```python
from build123d import *

# Parameters (mm, degrees)
BOSS_EXTRUDE1_DEPTH = 2
SKETCH2_R           = 1.5
CUT_EXTRUDE1_DEPTH  = 83.048765987
SKETCH3_R           = 1
CUT_EXTRUDE2_DEPTH  = 83.048765987


with BuildPart() as part:
    # Sketch1 → Boss-Extrude1 (new body)
    with BuildSketch(Plane(origin=(0, 0, 0), x_dir=(1, 0, 0), z_dir=(0, 1, 0))):
        with BuildLine():
            Line((53, 58), (-53, 58))
            ThreePointArc((-53, 58), (-56.535533906, 56.535533906), (-58, 53))
            Line((-58, 53), (-58, -53))
            ThreePointArc((-58, -53), (-56.535533906, -56.535533906), (-53, -58))
            Line((-53, -58), (53, -58))
            ThreePointArc((53, -58), (56.535533906, -56.535533906), (58, -53))
            Line((58, -53), (58, 53))
            ThreePointArc((58, 53), (56.535533906, 56.535533906), (53, 58))
        make_face()
    extrude(amount=BOSS_EXTRUDE1_DEPTH)

    # Sketch2 → Cut-Extrude1 (cut, through all)
    with BuildSketch(Plane(origin=(0, 2, 0), x_dir=(1, 0, 0), z_dir=(0, 1, 0))):
        with Locations(Location((-45.60494968, 43.386330507, 0), (0, 0, 270))):
            Circle(SKETCH2_R)
        with Locations(Location((-35.60494968, 43.386330507, 0), (0, 0, 270))):
            Circle(SKETCH2_R)
        with Locations(Location((-25.60494968, 43.386330507, 0), (0, 0, 270))):
            Circle(SKETCH2_R)
        with Locations(Location((-15.60494968, 43.386330507, 0), (0, 0, 270))):
            Circle(SKETCH2_R)
        with Locations(Location((-5.60494968, 43.386330507, 0), (0, 0, 270))):
            Circle(SKETCH2_R)
        with Locations(Location((4.39505032, 43.386330507, 0), (0, 0, 270))):
            Circle(SKETCH2_R)
        with Locations(Location((14.39505032, 43.386330507, 0), (0, 0, 270))):
            Circle(SKETCH2_R)
        with Locations(Location((24.39505032, 43.386330507, 0), (0, 0, 270))):
            Circle(SKETCH2_R)
        with Locations(Location((34.39505032, 43.386330507, 0), (0, 0, 270))):
            Circle(SKETCH2_R)
        with Locations(Location((44.39505032, 43.386330507, 0), (0, 0, 270))):
            Circle(SKETCH2_R)
        with Locations(Location((-35.60494968, 33.386330507, 0), (0, 0, 270))):
            Circle(SKETCH2_R)
        with Locations(Location((-25.60494968, 33.386330507, 0), (0, 0, 270))):
            Circle(SKETCH2_R)
        with Locations(Location((-15.60494968, 33.386330507, 0), (0, 0, 270))):
            Circle(SKETCH2_R)
        with Locations(Location((-5.60494968, 33.386330507, 0), (0, 0, 270))):
            Circle(SKETCH2_R)
        with Locations(Location((4.39505032, 33.386330507, 0), (0, 0, 270))):
            Circle(SKETCH2_R)
        with Locations(Location((14.39505032, 33.386330507, 0), (0, 0, 270))):
            Circle(SKETCH2_R)
        with Locations(Location((24.39505032, 33.386330507, 0), (0, 0, 270))):
            Circle(SKETCH2_R)
        with Locations(Location((34.39505032, 33.386330507, 0), (0, 0, 270))):
            Circle(SKETCH2_R)
        with Locations(Location((44.39505032, 33.386330507, 0), (0, 0, 270))):
            Circle(SKETCH2_R)
        with Locations(Location((-35.60494968, 23.386330507, 0), (0, 0, 270))):
            Circle(SKETCH2_R)
        with Locations(Location((-25.60494968, 23.386330507, 0), (0, 0, 270))):
            Circle(SKETCH2_R)
        with Locations(Location((-15.60494968, 23.386330507, 0), (0, 0, 270))):
            Circle(SKETCH2_R)
        with Locations(Location((-5.60494968, 23.386330507, 0), (0, 0, 270))):
            Circle(SKETCH2_R)
        with Locations(Location((4.39505032, 23.386330507, 0), (0, 0, 270))):
            Circle(SKETCH2_R)
        with Locations(Location((14.39505032, 23.386330507, 0), (0, 0, 270))):
            Circle(SKETCH2_R)
        with Locations(Location((24.39505032, 23.386330507, 0), (0, 0, 270))):
            Circle(SKETCH2_R)
        with Locations(Location((34.39505032, 23.386330507, 0), (0, 0, 270))):
            Circle(SKETCH2_R)
        with Locations(Location((44.39505032, 23.386330507, 0), (0, 0, 270))):
            Circle(SKETCH2_R)
        with Locations(Location((-35.60494968, 13.386330507, 0), (0, 0, 270))):
            Circle(SKETCH2_R)
        with Locations(Location((-25.60494968, 13.386330507, 0), (0, 0, 270))):
            Circle(SKETCH2_R)
        with Locations(Location((-15.60494968, 13.386330507, 0), (0, 0, 270))):
            Circle(SKETCH2_R)
        with Locations(Location((-5.60494968, 13.386330507, 0), (0, 0, 270))):
            Circle(SKETCH2_R)
        with Locations(Location((4.39505032, 13.386330507, 0), (0, 0, 270))):
            Circle(SKETCH2_R)
        with Locations(Location((14.39505032, 13.386330507, 0), (0, 0, 270))):
            Circle(SKETCH2_R)
        with Locations(Location((24.39505032, 13.386330507, 0), (0, 0, 270))):
            Circle(SKETCH2_R)
        with Locations(Location((34.39505032, 13.386330507, 0), (0, 0, 270))):
            Circle(SKETCH2_R)
        with Locations(Location((44.39505032, 13.386330507, 0), (0, 0, 270))):
            Circle(SKETCH2_R)
        with Locations(Location((-35.60494968, 3.386330507, 0), (0, 0, 270))):
            Circle(SKETCH2_R)
        with Locations(Location((-25.60494968, 3.386330507, 0), (0, 0, 270))):
            Circle(SKETCH2_R)
        with Locations(Location((-15.60494968, 3.386330507, 0), (0, 0, 270))):
            Circle(SKETCH2_R)
        with Locations(Location((-5.60494968, 3.386330507, 0), (0, 0, 270))):
            Circle(SKETCH2_R)
        with Locations(Location((4.39505032, 3.386330507, 0), (0, 0, 270))):
            Circle(SKETCH2_R)
        with Locations(Location((14.39505032, 3.386330507, 0), (0, 0, 270))):
            Circle(SKETCH2_R)
        with Locations(Location((24.39505032, 3.386330507, 0), (0, 0, 270))):
            Circle(SKETCH2_R)
        with Locations(Location((34.39505032, 3.386330507, 0), (0, 0, 270))):
            Circle(SKETCH2_R)
        with Locations(Location((44.39505032, 3.386330507, 0), (0, 0, 270))):
            Circle(SKETCH2_R)
        with Locations(Location((-35.60494968, -6.613669493, 0), (0, 0, 270))):
            Circle(SKETCH2_R)
        with Locations(Location((-25.60494968, -6.613669493, 0), (0, 0, 270))):
            Circle(SKETCH2_R)
        with Locations(Location((-15.60494968, -6.613669493, 0), (0, 0, 270))):
            Circle(SKETCH2_R)
        with Locations(Location((-5.60494968, -6.613669493, 0), (0, 0, 270))):
            Circle(SKETCH2_R)
        with Locations(Location((4.39505032, -6.613669493, 0), (0, 0, 270))):
            Circle(SKETCH2_R)
        with Locations(Location((14.39505032, -6.613669493, 0), (0, 0, 270))):
            Circle(SKETCH2_R)
        with Locations(Location((24.39505032, -6.613669493, 0), (0, 0, 270))):
            Circle(SKETCH2_R)
        with Locations(Location((34.39505032, -6.613669493, 0), (0, 0, 270))):
            Circle(SKETCH2_R)
        with Locations(Location((44.39505032, -6.613669493, 0), (0, 0, 270))):
            Circle(SKETCH2_R)
        with Locations(Location((-35.60494968, -16.613669493, 0), (0, 0, 270))):
            Circle(SKETCH2_R)
        with Locations(Location((-25.60494968, -16.613669493, 0), (0, 0, 270))):
            Circle(SKETCH2_R)
        with Locations(Location((-15.60494968, -16.613669493, 0), (0, 0, 270))):
            Circle(SKETCH2_R)
        with Locations(Location((-5.60494968, -16.613669493, 0), (0, 0, 270))):
            Circle(SKETCH2_R)
        with Locations(Location((4.39505032, -16.613669493, 0), (0, 0, 270))):
            Circle(SKETCH2_R)
        with Locations(Location((14.39505032, -16.613669493, 0), (0, 0, 270))):
            Circle(SKETCH2_R)
        with Locations(Location((24.39505032, -16.613669493, 0), (0, 0, 270))):
            Circle(SKETCH2_R)
        with Locations(Location((34.39505032, -16.613669493, 0), (0, 0, 270))):
            Circle(SKETCH2_R)
        with Locations(Location((44.39505032, -16.613669493, 0), (0, 0, 270))):
            Circle(SKETCH2_R)
        with Locations(Location((-35.60494968, -26.613669493, 0), (0, 0, 270))):
            Circle(SKETCH2_R)
        with Locations(Location((-25.60494968, -26.613669493, 0), (0, 0, 270))):
            Circle(SKETCH2_R)
        with Locations(Location((-15.60494968, -26.613669493, 0), (0, 0, 270))):
            Circle(SKETCH2_R)
        with Locations(Location((-5.60494968, -26.613669493, 0), (0, 0, 270))):
            Circle(SKETCH2_R)
        with Locations(Location((4.39505032, -26.613669493, 0), (0, 0, 270))):
            Circle(SKETCH2_R)
        with Locations(Location((14.39505032, -26.613669493, 0), (0, 0, 270))):
            Circle(SKETCH2_R)
        with Locations(Location((24.39505032, -26.613669493, 0), (0, 0, 270))):
            Circle(SKETCH2_R)
        with Locations(Location((34.39505032, -26.613669493, 0), (0, 0, 270))):
            Circle(SKETCH2_R)
        with Locations(Location((44.39505032, -26.613669493, 0), (0, 0, 270))):
            Circle(SKETCH2_R)
        with Locations(Location((-35.60494968, -36.613669493, 0), (0, 0, 270))):
            Circle(SKETCH2_R)
        with Locations(Location((-25.60494968, -36.613669493, 0), (0, 0, 270))):
            Circle(SKETCH2_R)
        with Locations(Location((-15.60494968, -36.613669493, 0), (0, 0, 270))):
            Circle(SKETCH2_R)
        with Locations(Location((-5.60494968, -36.613669493, 0), (0, 0, 270))):
            Circle(SKETCH2_R)
        with Locations(Location((4.39505032, -36.613669493, 0), (0, 0, 270))):
            Circle(SKETCH2_R)
        with Locations(Location((14.39505032, -36.613669493, 0), (0, 0, 270))):
            Circle(SKETCH2_R)
        with Locations(Location((24.39505032, -36.613669493, 0), (0, 0, 270))):
            Circle(SKETCH2_R)
        with Locations(Location((34.39505032, -36.613669493, 0), (0, 0, 270))):
            Circle(SKETCH2_R)
        with Locations(Location((44.39505032, -36.613669493, 0), (0, 0, 270))):
            Circle(SKETCH2_R)
        with Locations(Location((-35.60494968, -46.613669493, 0), (0, 0, 270))):
            Circle(SKETCH2_R)
        with Locations(Location((-25.60494968, -46.613669493, 0), (0, 0, 270))):
            Circle(SKETCH2_R)
        with Locations(Location((-15.60494968, -46.613669493, 0), (0, 0, 270))):
            Circle(SKETCH2_R)
        with Locations(Location((-5.60494968, -46.613669493, 0), (0, 0, 270))):
            Circle(SKETCH2_R)
        with Locations(Location((4.39505032, -46.613669493, 0), (0, 0, 270))):
            Circle(SKETCH2_R)
        with Locations(Location((14.39505032, -46.613669493, 0), (0, 0, 270))):
            Circle(SKETCH2_R)
        with Locations(Location((24.39505032, -46.613669493, 0), (0, 0, 270))):
            Circle(SKETCH2_R)
        with Locations(Location((34.39505032, -46.613669493, 0), (0, 0, 270))):
            Circle(SKETCH2_R)
        with Locations(Location((44.39505032, -46.613669493, 0), (0, 0, 270))):
            Circle(SKETCH2_R)
        with Locations(Location((-45.60494968, 33.386330507, 0), (0, 0, 270))):
            Circle(SKETCH2_R)
        with Locations(Location((-45.60494968, 23.386330507, 0), (0, 0, 270))):
            Circle(SKETCH2_R)
        with Locations(Location((-45.60494968, 13.386330507, 0), (0, 0, 270))):
            Circle(SKETCH2_R)
        with Locations(Location((-45.60494968, 3.386330507, 0), (0, 0, 270))):
            Circle(SKETCH2_R)
        with Locations(Location((-45.60494968, -6.613669493, 0), (0, 0, 270))):
            Circle(SKETCH2_R)
        with Locations(Location((-45.60494968, -16.613669493, 0), (0, 0, 270))):
            Circle(SKETCH2_R)
        with Locations(Location((-45.60494968, -26.613669493, 0), (0, 0, 270))):
            Circle(SKETCH2_R)
        with Locations(Location((-45.60494968, -36.613669493, 0), (0, 0, 270))):
            Circle(SKETCH2_R)
        with Locations(Location((-45.60494968, -46.613669493, 0), (0, 0, 270))):
            Circle(SKETCH2_R)
    extrude(amount=-CUT_EXTRUDE1_DEPTH, mode=Mode.SUBTRACT)

    # Sketch3 → Cut-Extrude2 (cut, through all)
    with BuildSketch(Plane.XZ):
        with Locations(Location((-53, 53, 0), (0, 0, 270))):
            Circle(SKETCH3_R)
        with Locations(Location((53, -53, 0), (0, 0, 270))):
            Circle(SKETCH3_R)
    extrude(amount=-CUT_EXTRUDE2_DEPTH, mode=Mode.SUBTRACT)


solid = part.part
```
The listing builds one solid part. Answer for the finished solid, in the listing's coordinates (mm). Give positions to 0.01 mm unless a question says otherwise; leave off trailing zeros. Answer as CSV lines item,"result". Start each with the question number.
Q1. Given pin 1 (1.8 mm diameter, centred on x = 24.4, z = -3.39, fed in from +Y), flat-ended and moving along its own axis, determine where the tip first touches the part or whether it passes through.
Q2. Determine the mould class of faces 1 (the cylindrical face through (-57, 1, 56)), 2 (the cylindrical face through (-26.518, 1.014, -14.577)) for opening direction Z: pulls with the +Z half, pulls with the -Z half, needs draft (parallel to the pull), parting line crosses it, or undercut.
Q3. A cutting plane is placed at A-A (y = 1.65). Count the separate pieces of the cut face and the enclosed holes in it, then the cut area to 3 significant figures.
Results found:
1,pin 1,"through"
2,face 1,"pulls with the +Z half"
2,face 2,"undercut"
3,separate pieces,"1"
3,enclosed holes,"102"
3,area,"12,700 mm2"
